Design review of the part shown in the three views and the two pictorial views. Dimensions are in mm from the part's minimum x, y and z. Round coordinates to 2 decimals unless told otherwise and drop trailing zeros. Loops run counter-clockwise (first coordinate to the right, second up) from the corner with the lowest first, then second, coordinate; pieces in that order, holes last. Notation, with made-up numbers: M 64,30.25 L 92,30.25 A16 ccw 92,46.25 Z; hole C 60,8.25 d5. An arc over 180 degrees is marked long. One line per question, with ' | ' between items. Start each with the question number.
1) We need section B-B (x = 4.5). Give the boundary of the cut face in (y, z).
2) For pin 1 Ø1 at (y, z) = (1.5, 16) entering from -X; pin 2 Ø1.5 at (x, y) = (9.5, 1.5) entering from +Z, all flat-tipped, find the tip position at first contact; note any pin that passes through.
3) We need section C-C (z = 8). Give the boundary of the cut face in (x, y).
4) For probe 1 along X at (y, z) = (2.8, 5) (1 decimal); probe 2 along Z at (x, y) = (5.75, 4.3); probe 3 along X at (y, z) = (1.4, 17) (1 decimal), list the stretches that pass through material, from the lowest coordinate up. Write a range as from..to.
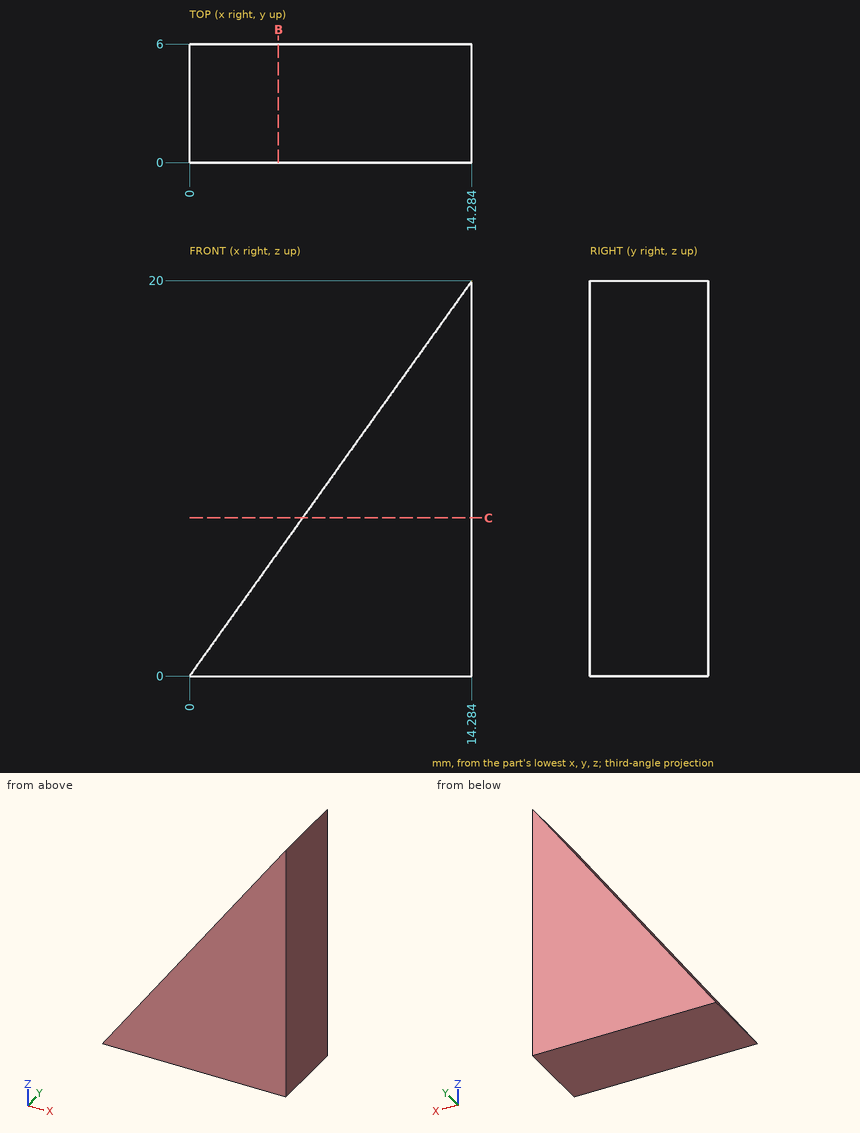
Answers below:
1) outline: M 0,0 L 6,0 L 6,6.3 L 0,6.3 Z
2) pin 1: x = 11.07 | pin 2: z = 14.35
3) outline: M 5.71,0 L 14.28,0 L 14.28,6 L 5.71,6 Z
4) probe 1: 3.6..14.3 | probe 2: 0..8.05 | probe 3: 12.1..14.3
